Can you work these out from the model? Positions are in its coordinate system, mm. Face numbers are marked on the shaded views. Round coordinates to 2 decimals unless told otherwise and drop trailing zeros. Loops run counter-clockwise (first coordinate to the right, second up) from the corner with the lowest first, then second, coordinate; pieces in that order, holes last. Notation, with made-up numbers: M 32,42.25 L 68,42.25 A17 ccw 68,74.25 Z; hole C 20,55.5 d3. An arc over 180 degrees is marked long. Return JSON: item names as keys, results as strings.
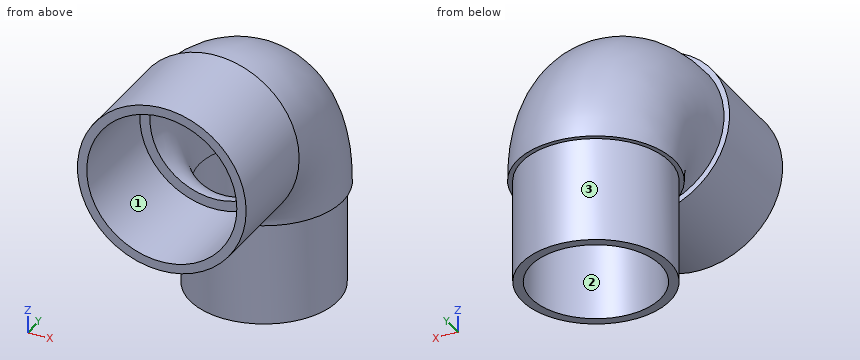
```python
from build123d import *

# Parameters (mm, degrees)
ESQUISSE1_R        = 16.9
ESQUISSE1_R_2      = 13.9
R_VOL_MINCE1_ANGLE = 90
ESQUISSE2_R        = 15.9
ESQUISSE2_R_2      = 13.9
EXTRU_MINCE1_DEPTH = 22.4
ESQUISSE3_R        = 18.1
ESQUISSE3_R_2      = 16.1
EXTRU_MINCE2_DEPTH = 22.3


with BuildPart() as part:
    # Esquisse1 → Révol.-Mince1 (revolve)
    with BuildSketch(Plane.XY):
        Circle(ESQUISSE1_R)
        Circle(ESQUISSE1_R_2, mode=Mode.SUBTRACT)
    revolve(axis=Axis((0, -20.745281933, 0), (1, 0, 0)), revolution_arc=R_VOL_MINCE1_ANGLE)

    # Esquisse2 → Extru.-Mince1 (add)
    with BuildSketch(Plane(origin=(0, 0, 0), x_dir=(-1, 0, 0), z_dir=(0, 0, -1))):
        Circle(ESQUISSE2_R)
        Circle(ESQUISSE2_R_2, mode=Mode.SUBTRACT)
    extrude(amount=EXTRU_MINCE1_DEPTH)

    # Esquisse3 → Extru.-Mince2 (add)
    with BuildSketch(Plane.XZ.offset(20.745281933)):
        with Locations((0, 20.745281933)):
            Circle(ESQUISSE3_R)
        with Locations((0, 20.745281933)):
            Circle(ESQUISSE3_R_2, mode=Mode.SUBTRACT)
    extrude(amount=EXTRU_MINCE2_DEPTH)


solid = part.part
```
Q1. Thinking about a two-plate mould opening in Y: for the marked faces 1, 2 and 3, which applies, pulls with the +Y half, pulls with the -Y half, needs draft (parallel to the pull), parting line crosses it, or undercut?
Results:
{"face 1": "needs draft", "face 2": "undercut", "face 3": "parting line crosses it"}
Q2. Suppose I cut it at A-A, the plane x = -6. Please give me the cut outline in (y, z), plus the area to 3 significant figures.
Results:
{"outline": "M -43.05,3.67 L -20.75,3.67 L -20.75,4.95 A4.95 cw -15.8,0 L -14.72,0 L -14.72,-22.4 L -12.54,-22.4 L -12.54,0 A8.21 ccw -20.75,8.21 L -20.75,5.81 L -43.05,5.81 Z; M -43.05,35.69 L -20.75,35.69 L -20.75,33.28 A33.28 cw 12.54,0 L 12.54,-22.4 L 14.72,-22.4 L 14.72,0 L 15.8,0 A36.54 ccw -20.75,36.54 L -20.75,37.82 L -43.05,37.82 Z", "area": "406 mm2"}
Q3. If I drill on line 1 along X through (y, z) = (-4, 13); line 2 along Y through (x, z) = (0, -11); line 3 along Z through (x, y) = (-10, -25), over which ranges is the centre line in solid material (lowest first)?
Results:
{"line 1": "x = -16.89 to -13.89, 13.89 to 16.89", "line 2": "y = -15.9 to -13.9, 13.9 to 15.9", "line 3": "z = 5.66 to 8.13, 33.36 to 35.83"}
Q4. Suppose I cut it at B-B, the plane z = -1.5. Please give me the cut outline in (x, y).
Results:
{"outline": "C 0,0 d31.8; hole C 0,0 d27.8"}
Q5. Suppose I cut it at C-C, the plane x = -0.5. Please give me the cut outline in (y, z), plus the area to 3 significant figures.
Results:
{"outline": "M -43.05,2.65 L -20.75,2.65 L -20.75,3.85 A3.85 cw -16.89,0 L -15.89,0 L -15.89,-22.4 L -13.89,-22.4 L -13.89,0 A6.85 ccw -20.75,6.85 L -20.75,4.65 L -43.05,4.65 Z; M -43.05,36.84 L -20.75,36.84 L -20.75,34.64 A34.64 cw 13.89,0 L 13.89,-22.4 L 15.89,-22.4 L 15.89,0 L 16.89,0 A37.64 ccw -20.75,37.64 L -20.75,38.84 L -43.05,38.84 Z", "area": "375 mm2"}
Q6. I'm going to push flat-ended pins straight in: pin 1 Ø1 at (x, z) = (3.5, 20) entering from -Y; pin 2 Ø6 at (x, z) = (3, 27.5) entering from -Y; pin 3 Ø8 at (x, y) = (-14, -10.5) entering from -Z; pin 4 Ø8 at (x, z) = (-12, 31.5) entering from +Y. Where does each tip first touch, or does it pass through?
Results:
{"pin 1": "stops at y = 6.59", "pin 2": "stops at y = -5.25", "pin 3": "stops at z = -22.4", "pin 4": "stops at y = -0.74"}
